from build123d import *

# Parameters (mm, degrees)
SKETCH1_W                = 22.5
SKETCH1_H                = 6.975
BOSS_EXTRUDE1_DEPTH      = 2.35
SKETCH2_R                = 1.475
BOSS_EXTRUDE2_DEPTH      = 8
SKETCH3_W                = 1.5
SKETCH3_H                = 6.975
BOSS_EXTRUDE3_DEPTH      = 3.85
SKETCH4_W                = 6.975
SKETCH4_H                = 3
BOSS_EXTRUDE4_DEPTH      = 3.5
SKETCH5_W                = 2.1
SKETCH5_H                = 6.975
CUT_EXTRUDE1_DEPTH       = 1.5
SKETCH6_R                = 1.05
BOSS_EXTRUDE5_DEPTH      = 6
BOSS_EXTRUDE9_DEPTH      = 7.76
BOSS_EXTRUDE9_DEPTH_BACK = 2.35
SKETCH7_R                = 2.4
FILLET1_R                = 2
FILLET2_R                = 2
FILLET3_R                = 1
FILLET4_DEPTH            = 2.35
FILLET5_R                = 1


with BuildPart() as part:
    # Sketch1 → Boss-Extrude1 (new body)
    with BuildSketch(Plane(origin=(0, 0, 0), x_dir=(1, 0, 0), z_dir=(0, 1, 0))):
        with Locations((-16.71505467, -8.920455339)):
            Rectangle(SKETCH1_W, SKETCH1_H)
    extrude(amount=BOSS_EXTRUDE1_DEPTH)

    # Sketch2 → Boss-Extrude2 (add)
    with BuildSketch(Plane(origin=(0, 2.35, 0), x_dir=(1, 0, 0), z_dir=(0, 1, 0))):
        with Locations(Location((-25.31505467, -10.457955339, 0), (0, 0, 270))):
            Circle(SKETCH2_R)
        with Locations(Location((-8.11505467, -10.457955339, 0), (0, 0, 270))):
            Circle(SKETCH2_R)
    extrude(amount=BOSS_EXTRUDE2_DEPTH)

    # Sketch3 → Boss-Extrude3 (add)
    with BuildSketch(Plane(origin=(0, 0, 0), x_dir=(-1, 0, 0), z_dir=(0, -1, 0))):
        with Locations((6.21505467, -8.920455339)):
            Rectangle(SKETCH3_W, SKETCH3_H)
    extrude(amount=BOSS_EXTRUDE3_DEPTH)

    # Sketch4 → Boss-Extrude4 (add)
    with BuildSketch(Plane(origin=(-5.46505467, 0, 0), x_dir=(0, 0, -1), z_dir=(1, 0, 0))):
        with Locations((-8.920455339, -2.35)):
            Rectangle(SKETCH4_W, SKETCH4_H)
    extrude(amount=BOSS_EXTRUDE4_DEPTH)

    # Sketch5 → Cut-Extrude1 (cut)
    with BuildSketch(Plane(origin=(0, -0.85, 0), x_dir=(1, 0, 0), z_dir=(0, 1, 0))):
        with Locations((-4.41505467, -8.920455339)):
            Rectangle(SKETCH5_W, SKETCH5_H)
    extrude(amount=-CUT_EXTRUDE1_DEPTH, mode=Mode.SUBTRACT)

    # Sketch6 → Boss-Extrude5 (add)
    with BuildSketch(Plane(origin=(0, 2.35, 0), x_dir=(1, 0, 0), z_dir=(0, 1, 0))):
        with Locations(Location((-7.76505467, -7.007955339, 0), (0, 0, 270))):
            Circle(SKETCH6_R)
        with Locations(Location((-25.66505467, -7.007955339, 0), (0, 0, 270))):
            Circle(SKETCH6_R)
    extrude(amount=BOSS_EXTRUDE5_DEPTH)

    # Sketch7 → Boss-Extrude9 (add, two sides: drawn at the far end of the back side and taken through both)
    with BuildSketch(Plane(origin=(0, 0, 0), x_dir=(-1, 0, 0), z_dir=(0, -1, 0)).offset(-BOSS_EXTRUDE9_DEPTH_BACK)):
        with Locations(Location((16.71505467, -14.367955339, 0), (0, 0, 90))):
            Circle(SKETCH7_R)
        with Locations(Location((24.68505467, -14.367955339, 0), (0, 0, 90))):
            Circle(SKETCH7_R)
    extrude(amount=BOSS_EXTRUDE9_DEPTH + BOSS_EXTRUDE9_DEPTH_BACK)

    # Fillet1
    fillet1_edges = [part.edges().sort_by_distance(p)[0] for p in [
        (-6.96505467, -3.85, 8.920455339),
    ]]
    fillet(fillet1_edges, radius=FILLET1_R)

    # Fillet2
    fillet2_edges = [part.edges().sort_by_distance(p)[0] for p in [
        (-1.96505467, -3.85, 8.920455339),
    ]]
    fillet(fillet2_edges, radius=FILLET2_R)

    # Fillet3
    fillet3_edges = [part.edges().sort_by_distance(p)[0] for p in [
        (-1.96505467, -0.85, 8.920455339),
    ]]
    fillet(fillet3_edges, radius=FILLET3_R - 0.0001)  # a hair under: the kernel refuses the full size

    # Fillet4: read off the stored shape, not the designer's step
    # Fillet4 outline → Fillet4 (add)
    with BuildSketch(Plane(origin=(0, 0, 0), x_dir=(1, 0, 0), z_dir=(0, 1, 0))):
        with BuildLine():
            add(Edge.make_bspline(
                [(-7.274800436, -12.407955339), (-11.89332012, -12.407955339), (-14.887908689, -15.924084371)],
                knots=[0, 0, 0, 1, 1, 1], degree=2, weights=[1, 0.907851061, 1]))
            Line((-7.274800436, -12.407955339), (-15.329991494, -12.407955339))
            ThreePointArc((-15.329991494, -12.407955339), (-14.333802319, -14.068560547), (-14.887908689, -15.924084371))
        make_face()
        with BuildLine():
            add(Edge.make_bspline(
                [(-18.54220065, -15.924084371), (-19.483433236, -14.818925802), (-20.700054672, -14.027012596)],
                knots=[0, 0, 0, 0.335510555, 0.335510555, 0.335510555], degree=2, weights=[1, 0.969083058, 0.958912037]))
            ThreePointArc((-18.54220065, -15.924084371), (-19.096307021, -14.068560547), (-18.100117845, -12.407955339))
            Line((-18.100117845, -12.407955339), (-23.299991494, -12.407955339))
            ThreePointArc((-23.299991494, -12.407955339), (-22.303802319, -14.068560547), (-22.857908689, -15.924084371))
            add(Edge.make_bspline(
                [(-20.700054672, -14.027012596), (-21.916676104, -14.818925803), (-22.857908689, -15.924084371)],
                knots=[0.664489445, 0.664489445, 0.664489445, 1, 1, 1], degree=2, weights=[0.958912037, 0.969083058, 1]))
        make_face()
        with BuildLine():
            ThreePointArc((-27.023832507, -14.906581581), (-26.92727037, -13.512111455), (-26.070117845, -12.407955339))
            Line((-26.070117845, -12.407955339), (-27.96505467, -12.407955339))
            add(Edge.make_bspline(
                [(-27.023832507, -14.906581581), (-27.326152305, -13.59387383), (-27.96505467, -12.407955339)],
                knots=[0, 0, 0, 1, 1, 1], degree=2, weights=[1, 0.991048646, 1]))
        make_face()
    extrude(amount=FILLET4_DEPTH)

    # Fillet5
    fillet5_edges = [part.edges().sort_by_distance(p)[0] for p in [
        (-20.700054672, 1.175, 14.027012596),
    ]]
    fillet(fillet5_edges, radius=FILLET5_R)


solid = part.part
The listing builds one solid part. Answer for the finished solid, in the listing's coordinates (mm). A direction names the side the tool comes from. Coordinates: 2 decimals unless noted, no trailing zeros. Write each loop counter-clockwise with the first axis right and the second up, starting at its lowest first coordinate (ties: lowest second). Pieces come first, ordered by that corner, then holes. Notation, with made-up numbers: (-37, 88.25) - (-18, 88.25) arc R22 ccw to (-18, 107.25) - close; hole circle Ø7 at (15, -23.75). An arc over 180 degrees is marked (long way). Return JSON: item names as keys, results as strings.
1. Which of the six approach directions +Z, -Z, +X, -X, +Y, -Y give full straight-line access (tool end or side, diameter ignored) to faces 5 (the face through (-8.167, 5.308, 7.978)), 6 (the face through (-8, 8.35, 7)), 7 (the face through (-24.58, -3.758, 16.766))?
Final values:
{"face 5": "+Y", "face 6": "-Z, +X, -X, +Y", "face 7": "-Y"}
2. Each of these flat-tipped pins is pushed along its axis until it touches: pin 1 Ø1.7 at (x, z) = (-7.5, 7.5) entering from +Y; pin 2 Ø3 at (y, z) = (5.5, 10) entering from -X; pin 3 Ø3.5 at (x, z) = (-22, 10.5) entering from +Y. Where does it stop, or does it pass through?
Final values:
{"pin 1": "y = 8.35", "pin 2": "x = -26.79", "pin 3": "y = 2.35"}
3. The part is cut by section A-A on y = -3. Determine the outline of the cut face in (x, z), then the cut area to 3 significant figures.
Final values:
{"outline": "circle Ø4.8 at (-24.69, 14.37); circle Ø4.8 at (-16.72, 14.37); (-6.6, 5.43) - (-2.33, 5.43) - (-2.33, 12.41) - (-6.6, 12.41) - close", "area": "66.0 mm^2"}
4. Consider line 1 along Y through (x, z) = (-23, 8.75); line 2 along X through (y, z) = (-0.75, 6.5); line 3 along X through (y, z) = (1.25, 11.5). Determine where each line is inside the solid, lowest interval first.
Final values:
{"line 1": "0 to 2.35", "line 2": "-6.97 to -5.47", "line 3": "-27.97 to -5.47"}
5. For a pull along X with two mould halves and no side action, classify faces 1 (the face through (-17, -7.76, 14)), 2 (the face through (-16.61, -3.758, 16.766)), 3 (the face through (-5.465, 0, 9)), 4 (the face through (-2.566, -3.28, 8.872)) as +X half, -X half, draft (parallel to the pull), parting line (faces both ways), or undercut.
Final values:
{"face 1": "draft", "face 2": "undercut", "face 3": "undercut", "face 4": "+X half"}
6. The part is cut by section C-C on y = 3.25. Determine the outline of the cut face in (x, z) (3 decimals), then the cut area to 3 significant figures.
Final values:
{"outline": "circle Ø2.95 at (-25.315, 10.458); circle Ø2.1 at (-25.665, 7.008); circle Ø2.95 at (-8.115, 10.458); circle Ø2.1 at (-7.765, 7.008)", "area": "20.6 mm^2"}
